Part print with two shaded views. Sizes in mm from the minimum x, y, z corner. A direction names the side the tool comes from. Coordinates: 2 decimals unless noted, no trailing zeros. Write each loop counter-clockwise with the first axis right and the second up, starting at its lowest first coordinate (ties: lowest second). Pieces come first, ordered by that corner, then holes. Notation, with made-up numbers: M 70,-31.5 L 91,-31.5 A29 cw 91,-6.5 Z; hole C 38,-19.75 d4. An arc over 180 degrees is marked long. Answer in a Markdown table with one row per item. Add a question column.
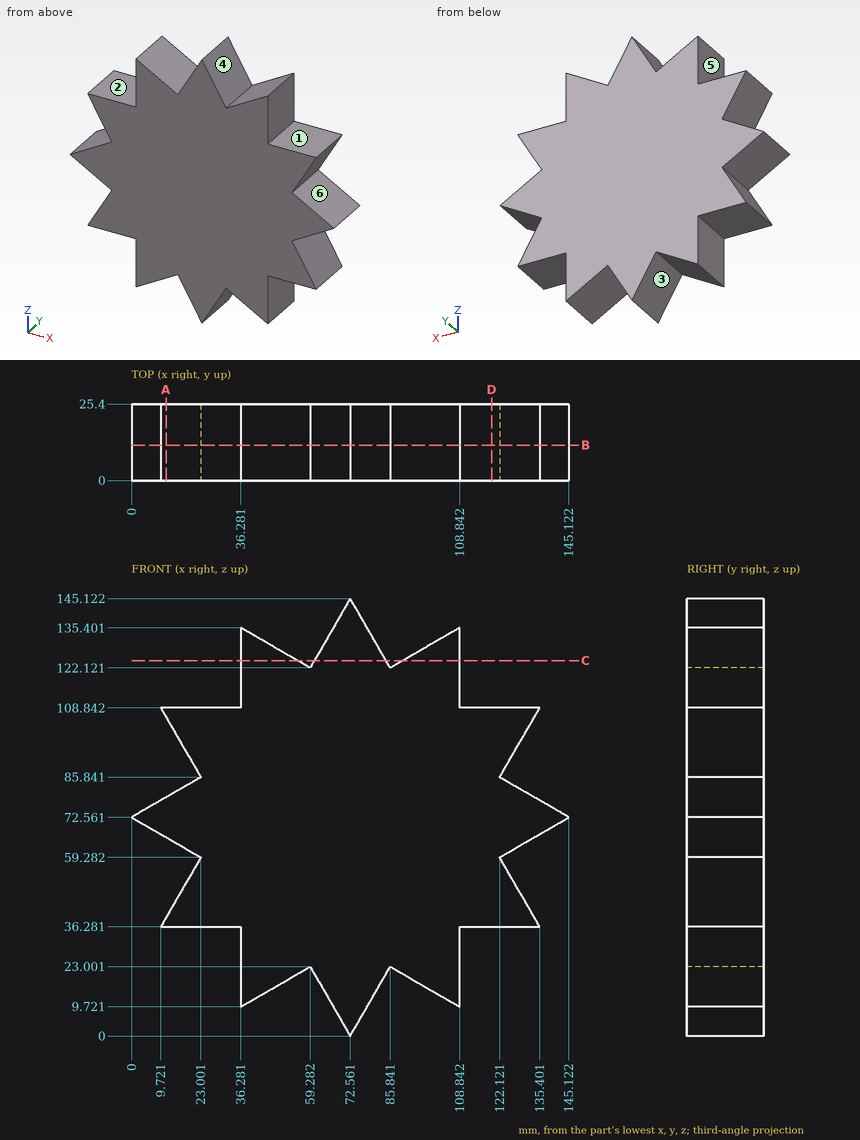
1) Slice it at C-C (z = 124.5). Give the cut face in (x, y) (1 decimal), then the cut area to 3 significant figures.
2) Slice it at B-B (y = 11.75). Give the cut face in (x, z), then the cut area to 3 significant figures.
3) Two-plate mould, pull along X, no slides. Class the marked faces 4, 5 and 6: released by +X, released by -X, zero draft, split by the parting line, or undercut.
4) Slice it at A-A (x = 11.5). Give the cut face in (y, z).
5) Which spindle directions (+Z, -Z, +X, -X, +Y, -Y) get a long thin tool onto all of the face, cutting with end or side? Do the marked faces 1, 2 and 3. Say none if no direction does.
6) Flat gauge pins, fed straight in: pin 1 Ø7.5 at (y, z) = (16, 19) entering from +X; pin 2 Ø5 at (x, y) = (52, 14.5) entering from +Z; pin 3 Ø5 at (x, y) = (91, 6.5) entering from +Z. Where does each tip first touch, or does it go through?
7) Slice it at D-D (x = 119.5). Give the cut face in (y, z), then the cut area to 3 significant figures.
8) Drill centre lines: probe 1 along X at (y, z) = (22, 123) (1 decimal); probe 2 along X at (y, z) = (14.5, 120.5); probe 3 along X at (y, z) = (15.75, 12) (1 decimal). Where is each one in solid material? Low to high.
Ans:
| question | item | result |
|---|---|---|
| 1 | outline | M 36.3,0 L 55.2,0 L 55.2,25.4 L 36.3,25.4 Z; M 60.7,0 L 84.5,0 L 84.5,25.4 L 60.7,25.4 Z; M 90,0 L 108.8,0 L 108.8,25.4 L 90,25.4 Z |
| 1 | area | 1,560 mm2 |
| 2 | outline | M 0,72.56 L 23,59.28 L 9.72,36.28 L 36.28,36.28 L 36.28,9.72 L 59.28,23 L 72.56,0 L 85.84,23 L 108.84,9.72 L 108.84,36.28 L 135.4,36.28 L 122.12,59.28 L 145.12,72.56 L 122.12,85.84 L 135.4,108.84 L 108.84,108.84 L 108.84,135.4 L 85.84,122.12 L 72.56,145.12 L 59.28,122.12 L 36.28,135.4 L 36.28,108.84 L 9.72,108.84 L 23,85.84 Z |
| 2 | area | 11,600 mm2 |
| 3 | face 4 | undercut |
| 3 | face 5 | released by -X |
| 3 | face 6 | released by +X |
| 4 | outline | M 0,36.28 L 25.4,36.28 L 25.4,39.36 L 0,39.36 Z; M 0,65.92 L 25.4,65.92 L 25.4,79.2 L 0,79.2 Z; M 0,105.76 L 25.4,105.76 L 25.4,108.84 L 0,108.84 Z |
| 5 | face 1 | +Z, +X, +Y, -Y |
| 5 | face 2 | +Z, -X, +Y, -Y |
| 5 | face 3 | -Z, +Y, -Y |
| 6 | pin 1 | stops at x = 108.84 |
| 6 | pin 2 | stops at z = 127.77 |
| 6 | pin 3 | stops at z = 126.54 |
| 7 | outline | M 0,36.28 L 25.4,36.28 L 25.4,108.84 L 0,108.84 Z |
| 7 | area | 1,840 mm2 |
| 8 | probe 1 | x = 36.3 to 57.8, 59.8 to 85.3, 87.4 to 108.8 |
| 8 | probe 2 | x = 36.28 to 108.84 |
| 8 | probe 3 | x = 36.3 to 40.2, 65.6 to 79.5, 104.9 to 108.8 |
